Could you check a few things on this model? Use its own coordinates, in mm. A direction names the side the tool comes from. Give positions to 0.01 mm unless a question says otherwise; leave off trailing zeros. Write each loop counter-clockwise with the first axis right and the second up, starting at its lowest first coordinate (ties: lowest second). Pieces come first, ordered by that corner, then holes. Notation, with made-up numbers: (2.25, -23) -> (30.25, -23) arc R18 ccw to (30.25, -12) -> close; hole circle Ø1 at (32.25, 60.5). An arc over 180 degrees is marked (long way). Write item = value, one per line. Start each with the question number.
```python
from build123d import *

# Parameters (mm, degrees)
F1_DEPTH = 30
F3_D     = 4.2
F3_DEPTH = 8
F3_TIP   = 1.2618073
F6_DEPTH = 20


with BuildPart() as f1:
    # F0 (on Front) → F1 (new body)
    with BuildSketch(Plane.XZ):
        Polygon((-10, 0), (10, 0), (10, 6), (5, 11), (10, 16), (10, 17.5), (7.5, 17.5), (7.5, 20), (-10, 20), align=None)
    extrude(amount=F1_DEPTH)

    # F3
    with Locations(Plane(origin=(0, 0, 0), x_dir=(1, 0, 0), z_dir=(0, 0, -1))):
        with Locations((0, 15)):
            Hole(F3_D / 2, depth=F3_DEPTH)
            with Locations((0, 0, -(F3_DEPTH + F3_TIP / 2))):  # 118° drill point
                Cone(0, F3_D / 2, F3_TIP, mode=Mode.SUBTRACT)

    # F4: F1 across plane


with BuildPart() as f1_1:
    add(f1.part)
    add(f1.part.mirror(Plane.XZ))

    # F5 (on Top) → F6 (cut, through all)
    with BuildSketch(Plane.XY):
        Polygon((10, 4), (6, 0), (10, -4), align=None)
    extrude(amount=F6_DEPTH, mode=Mode.SUBTRACT)


solid = f1_1.part
```
(1) Imagine slicing it at C-C (y = 22.5). Please give me the cut outline in (x, z), then the cut area to 3 significant figures.
(2) I'm going to push a flat-ended pin straight in: pin 1 (2.5 mm diameter, centred on x = 0, y = 15, fed in from -Z). Where does the tip first touch, or does it pass through?
(3) On a 3-axis mill with a long thin cutter (end or side, diameter ignored), from which of +Z, -Z, +X, -X, +Y, -Y can I reach the whole of each face in a straight line? I mean faces 1 (the flat face through (5.9, -0.4, 10.1)), 2 (the flat face through (9, 16, 17.5)), 3 (the cylindrical face through (0.273, 17.082, 4.056)). Say none if no direction works.
(4) If I drill on line 1 along Y through (x, z) = (0, 5); line 2 along X through (y, z) = (-15, 6); line 3 along Y through (x, z) = (1, 5.25), over which ranges is the centre line in solid material (lowest first)? Write a range as from..to.
(5) Imagine slicing it at D-D (z = 15). Please give me the cut outline in (x, y), then the cut area to 3 significant figures.
(6) We'd pull the mould along Z, two halves only. Please class faces 4 (the flat face through (9, -16, 17.5)), 5 (the flat face through (8, -2, 16)), 6 (the flat face through (5.8, -0.4, 11.8)): released by +Z, released by -Z, zero draft, split by the parting line, or undercut.
(7) Imagine slicing it at B-B (z = 2). Please give me the cut outline in (x, y), then the cut area to 3 significant figures.
(8) Imagine slicing it at A-A (x = 8.25). Please give me the cut outline in (y, z), then the cut area to 4 significant figures.
Answers below:
q1.outline = (-10, 0) -> (10, 0) -> (10, 6) -> (5, 11) -> (10, 16) -> (10, 17.5) -> (7.5, 17.5) -> (7.5, 20) -> (-10, 20) -> close
q1.area = 369 mm^2
q2.pin_1 = 8.51
q3.face_1 = +X, +Y, -Y
q3.face_2 = +Z, +X, +Y, -Y
q3.face_3 = -Z
q4.line_1 = -30..-17.1, -12.9..12.9, 17.1..30
q4.line_2 = -10..-2.1, 2.1..10
q4.line_3 = -30..-16.85, -13.15..13.15, 16.85..30
q5.outline = (-10, -30) -> (9, -30) -> (9, -3) -> (6, 0) -> (9, 3) -> (9, 30) -> (-10, 30) -> close
q5.area = 1,130 mm^2
q6.face_4 = released by +Z
q6.face_5 = zero draft
q6.face_6 = undercut
q7.outline = (-10, -30) -> (10, -30) -> (10, -4) -> (6, 0) -> (10, 4) -> (10, 30) -> (-10, 30) -> close; hole circle Ø4.2 at (0, -15); hole circle Ø4.2 at (0, 15)
q7.area = 1,160 mm^2
q8.outline = (-30, 0) -> (-2.25, 0) -> (-2.25, 7.75) -> (-30, 7.75) -> close; (-30, 14.25) -> (-2.25, 14.25) -> (-2.25, 17.5) -> (-30, 17.5) -> close; (2.25, 0) -> (30, 0) -> (30, 7.75) -> (2.25, 7.75) -> close; (2.25, 14.25) -> (30, 14.25) -> (30, 17.5) -> (2.25, 17.5) -> close
q8.area = 610.5 mm^2
